Build history of the part. All positions in model axes, mm. A direction names the side the tool comes from. Give positions to 0.01 mm unless a question says otherwise; leave off trailing zeros. Loops run counter-clockwise (first coordinate to the right, second up) from the corner with the lowest first, then second, coordinate; pieces in that order, holes last. Notation, with made-up numbers: (1.25, 70.5) - (43.25, 70.5) arc R25 ccw to (43.25, 100.5) - close; hole circle Ø6 at (51, 37.5). An arc over 180 degrees is marked (long way). Return JSON: item names as keys, results as strings. Group by question number.
1) Slice it at D-D (z = 4.35). Count the separate pieces of the cut face and the enclosed holes in it, and give its area (3 significant figures).
2) Drop flat-ended pins along their axis: pin 1 (1.2 mm diameter, centred on y = 11, z = 2, fed in from -X); pin 2 (2.5 mm diameter, centred on x = 15.5, y = 101.3, fed in from -Z). Give the stop position or say it passes through.
3) Mould opens along X. For faces 3 (the face through (47, 81, 3)), 4 (the face through (1, 63, 6)), 5 (the face through (-0.397, 148.824, 2.958)) say: released by +X, released by -X, zero draft, split by the parting line, or undercut.
4) Slice it at C-C (x = -12). List the corners of the cut face in (y, z), and give its area (3 significant figures).
5) Drill centre lines: probe 1 along X at (y, z) = (145.8, 2); probe 2 along Y at (x, z) = (-36, 3.85); probe 3 along X at (y, z) = (120, 4.75). Where is each one in solid material? Low to high. Write a range as from..to.
6) 3-axis set-ups, long thin cutter, end or side, ignore diameter. For faces 1 (the face through (0, 132.7, 3)), 2 (the face through (43.39, 156.58, 2.96)): which of +Z, -Z, +X, -X, +Y, -Y reach the whole face in a straight line?
7) Slice it at A-A (y = 145.8). List the corners of the cut face in (x, z), and give its area (3 significant figures).
8) Slice it at B-B (y = 85.8). List the corners of the cut face in (x, z).
```python
from build123d import *

# Parameters (mm, degrees)
MODEL_R                         = 16
MODEL_R_2                       = 3.05
MODEL_R_3                       = 2.6
MODEL_W                         = 13.5
MODEL_H                         = 6.2
BASE_DEPTH                      = 6
SKETCH1_R                       = 1.75
SENSORMOUNT_DEPTH               = 167.868211472
SKETCH2_R                       = 1.75
CABLEMOUNT_DEPTH                = 10
FILLETCABLESLOT_R               = 2
F_3_2_3_2_STEPPER_MOUNT_HOLES_D = 3.2


with BuildPart() as part:
    # Model → Base (new body)
    with BuildSketch(Plane.XY):
        with BuildLine():
            Line((-35, 160), (35, 160))
            ThreePointArc((35, 160), (43.485281374, 156.485281374), (47, 148))
            Line((47, 148), (47, 12))
            ThreePointArc((47, 12), (43.485281374, 3.514718626), (35, 0))
            Line((35, 0), (-35, 0))
            ThreePointArc((-35, 0), (-43.485281374, 3.514718626), (-47, 12))
            Line((-47, 12), (-47, 148))
            ThreePointArc((-47, 148), (-43.485281374, 156.485281374), (-35, 160))
        make_face()
        with Locations((0, 85.8)):
            Circle(MODEL_R, mode=Mode.SUBTRACT)
        with Locations((0, 145.8)):
            Circle(MODEL_R_2, mode=Mode.SUBTRACT)
        with Locations((-20, 145.8)):
            Circle(MODEL_R_3, mode=Mode.SUBTRACT)
        with Locations((20, 145.8)):
            Circle(MODEL_R_3, mode=Mode.SUBTRACT)
        with Locations((-35, 70.45)):
            Circle(MODEL_R_3, mode=Mode.SUBTRACT)
        with Locations((0, 125.8)):
            Circle(MODEL_R_2, mode=Mode.SUBTRACT)
        with Locations((35, 70.45)):
            Circle(MODEL_R_3, mode=Mode.SUBTRACT)
        with BuildLine():
            Line((-32.4, 12.5), (-32.4, 10))
            ThreePointArc((-32.4, 10), (-35, 7.4), (-37.6, 10))
            Line((-37.6, 10), (-37.6, 12.5))
            ThreePointArc((-37.6, 12.5), (-35, 15.1), (-32.4, 12.5))
        make_face(mode=Mode.SUBTRACT)
        with BuildLine():
            Line((32.4, 12.5), (32.4, 10))
            ThreePointArc((32.4, 10), (35, 7.4), (37.6, 10))
            Line((37.6, 10), (37.6, 12.5))
            ThreePointArc((37.6, 12.5), (35, 15.1), (32.4, 12.5))
        make_face(mode=Mode.SUBTRACT)
        with Locations((0, 135.8)):
            Rectangle(MODEL_W, MODEL_H, mode=Mode.SUBTRACT)
    extrude(amount=BASE_DEPTH)

    # Sketch1 → SensorMount (cut, through all)
    with BuildSketch(Plane.XY.offset(6)):
        with Locations((-33, 120)):
            Circle(SKETCH1_R)
        with Locations((-33, 112.5)):
            Circle(SKETCH1_R)
    extrude(amount=-SENSORMOUNT_DEPTH, mode=Mode.SUBTRACT)

    # Sketch2 → CableMount (cut)
    with BuildSketch(Plane.XY.offset(6)):
        with Locations((22.5, 50.76)):
            Circle(SKETCH2_R)
        with Locations((31, 50.76)):
            Circle(SKETCH2_R)
    extrude(amount=-CABLEMOUNT_DEPTH, mode=Mode.SUBTRACT)

    # FilletCableSlot
    filletcableslot_edges = [part.edges().sort_by_distance(p)[0] for p in [
        (6.75, 138.9, 3),
        (-6.75, 138.9, 3),
        (-6.75, 132.7, 3),
        (6.75, 132.7, 3),
    ]]
    fillet(filletcableslot_edges, radius=FILLETCABLESLOT_R)

    # Ø3.2 (3.2) Stepper mount Holes (through all)
    with Locations(Plane.XY.offset(6)):
        with Locations((-15.5, 101.3), (-15.5, 70.3), (15.5, 70.3), (15.5, 101.3)):
            Hole(F_3_2_3_2_STEPPER_MOUNT_HOLES_D / 2)


solid = part.part
```
Results:
{
 "1": {"separate pieces": "1", "enclosed holes": "18", "area": "13,700 mm2"},
 "2": {"pin 1": "x = -46.99", "pin 2": "through"},
 "3": {"face 3": "released by +X", "face 4": "zero draft", "face 5": "undercut"},
 "4": {"outline": "(0, 0) - (75.22, 0) - (75.22, 6) - (0, 6) - close; (96.38, 0) - (160, 0) - (160, 6) - (96.38, 6) - close", "area": "833 mm2"},
 "5": {"probe 1": "-47..-22.6, -17.4..-3.05, 3.05..17.4, 22.6..47", "probe 2": "0.04..7.6, 14.9..68.05, 72.85..159.96", "probe 3": "-47..-34.75, -31.25..47"},
 "6": {"face 1": "+Z, -Z", "face 2": "+Z, -Z, +X, +Y"},
 "7": {"outline": "(-47, 0) - (-22.6, 0) - (-22.6, 6) - (-47, 6) - close; (-17.4, 0) - (-3.05, 0) - (-3.05, 6) - (-17.4, 6) - close; (3.05, 0) - (17.4, 0) - (17.4, 6) - (3.05, 6) - close; (22.6, 0) - (47, 0) - (47, 6) - (22.6, 6) - close", "area": "465 mm2"},
 "8": {"outline": "(-47, 0) - (-16, 0) - (-16, 6) - (-47, 6) - close; (16, 0) - (47, 0) - (47, 6) - (16, 6) - close"}
}
